Input: part model. Units: mm. Frame: model coordinates. A direction names the side the tool comes from. Coordinates: 2 decimals unless noted, no trailing zeros. Loops run counter-clockwise (first coordinate to the right, second up) from the corner with the lowest first, then second, coordinate; pieces in that order, holes last. Notation, with made-up numbers: (35.25, -2.5) - (81.25, -2.5) arc R17 ccw to (81.25, 10.5) - close; hole circle Ø5 at (51.5, 28). An arc over 180 degrees is marked (long way). Use a Markdown table: item, result. Add a question column.
1. Section query A-A on z = 0. Return the cut outline in (x, y).
2. Section query C-C on z = 3. Return the cut outline in (x, y).
3. Section query D-D on y = 6. State how many separate pieces and enclosed holes the cut face has, then the cut area to 3 significant figures.
4. Ray query, L1, parallel to X at y = 12, z = 0; L2, parallel to Z at x = -26, y = 10.5; L3, parallel to X at y = 9.5, z = -2. Return the intervals inside material, ascending. Write a range as [from, to].
5. Contact query for flat-ended pins moving along their axis: P1, Ø3, axis at y = 3, z = 4, coming from the +X side; P2, Ø6, axis at x = -11, y = 11, coming from the -Z side; P3, Ø1, axis at x = 8, z = 10.5, coming from the -Y side. Output: stop coordinate, or through.
6. Draft query along X for faces 6 (the face through (23.69, 2.6, 8.61)), 7 (the face through (0, 20, 10)), 8 (the face through (26.9, 9.9, -3.4)). Return one class per face: released by +X, released by -X, zero draft, split by the parting line, or undercut.
7. Section query B-B on x = -4.5. Return the cut outline in (y, z), then the cut area to 3 significant figures.
8. Access query for faces 1 (the face through (26.165, 2.867, 5.156)), 2 (the face through (15.671, 10.337, 11.355)), 3 (the face through (26, 0, 4)), 4 (the face through (25, 1.996, 7)), 5 (the face through (-26.73, 9.86, -3.39)). Directions: +Z, -Z, +X, -X, +Y, -Y. A direction counts if a zero-diameter tool reaches every point of the face in a straight line with its end or side. Return the directions, or none.
```python
from build123d import *

# Parameters (mm, degrees)
SKETCH_1_R               = 2.2
EXTRUDE_1_DEPTH          = 20
FILLET_1_R               = 3
SKETCH_3_W               = 5.163325916
SKETCH_3_H               = 16.003609002
CUT_EXTRUDE_2_DEPTH      = 57.596101085
FILLET_2_R               = 2
EXTRUDE_2_DEPTH          = 20
CUT_EXTRUDE_1_DEPTH      = 40.134639439
CUT_EXTRUDE_1_DEPTH_BACK = 40.134639439
SKETCH_5_W               = 17
SKETCH_5_H               = 15.6
SKETCH_5_W_2             = 3.540430575
SKETCH_5_H_2             = 6.8
CUT_EXTRUDE_3_DEPTH      = 0.4
FILLET_3_R               = 1.5


with BuildPart() as part:
    # 草图1 → 凸台-拉伸1 (new body)
    with BuildSketch(Plane(origin=(0, 0, 0), x_dir=(1, 0, 0), z_dir=(0, 1, 0))):
        with BuildLine():
            Line((-29.65627848, -2.122306442), (-22.56320207, -11))
            Line((-22.56320207, -11), (22.56320207, -11))
            Line((22.56320207, -11), (29.65627848, -2.122306442))
            ThreePointArc((29.65627848, -2.122306442), (25.48101359, 3.04182187), (27.10063693, -3.398510293))
            Line((27.10063693, -3.398510293), (21.985991405, -9.8))
            Line((21.985991405, -9.8), (-21.985991405, -9.8))
            Line((-21.985991405, -9.8), (-27.10063693, -3.398510293))
            ThreePointArc((-27.10063693, -3.398510293), (-25.48101359, 3.04182187), (-29.65627848, -2.122306442))
        make_face()
        with Locations(Location((-27, 0, 0), (0, 0, 270))):
            Circle(SKETCH_1_R, mode=Mode.SUBTRACT)
        with Locations(Location((27, 0, 0), (0, 0, 90))):
            Circle(SKETCH_1_R, mode=Mode.SUBTRACT)
    extrude(amount=EXTRUDE_1_DEPTH)

    # 圆角1
    fillet_1_edges = [part.edges().sort_by_distance(p)[0] for p in [
        (-27.10063693, 10, 3.398510293),
        (27.10063693, 10, 3.398510293),
    ]]
    fillet(fillet_1_edges, radius=FILLET_1_R)

    # 草图3 → 切除-拉伸2 (cut, through all)
    with BuildSketch(Plane(origin=(19.136124058, 0, 15.289330416), x_dir=(0.6242077770989366, 0, -0.7812583766009837), z_dir=(0.7812583766009837, 0, 0.6242077770989366))):
        with Locations((10.071947024, 9.998195499)):
            Rectangle(SKETCH_3_W, SKETCH_3_H)
    cut_extrude_2 = extrude(amount=-CUT_EXTRUDE_2_DEPTH, mode=Mode.SUBTRACT)

    # 镜向1: 切除-拉伸2 across plane
    add(cut_extrude_2.mirror(Plane(origin=(0, 0, 0), x_dir=(0, 0, 1), z_dir=(1, 0, 0))), mode=Mode.SUBTRACT)

    # 圆角2
    fillet_2_edges = [part.edges().sort_by_distance(p)[0] for p in [
        (23.342862598, 1.996390998, 9.062958581),
        (26.211335217, 18, 4.745817031),
        (26.211335217, 1.996390998, 4.745817031),
        (23.342862598, 18, 9.062958581),
        (-23.342862598, 18, 9.062958581),
        (-26.211335217, 1.996390998, 4.745817031),
        (-26.211335217, 18, 4.745817031),
        (-23.342862598, 1.996390998, 9.062958581),
    ]]
    fillet(fillet_2_edges, radius=FILLET_2_R)

    # 草图4 → 凸台-拉伸2 (add)
    with BuildSketch(Plane(origin=(0, 20, 0), x_dir=(1, 0, 0), z_dir=(0, 1, 0))):
        Polygon((-22.56320207, -11), (-22.003917898, -11.7), (-16.284224925, -11.7), (-15.040430575, -11), align=None)
        Polygon((15.040430575, -11), (22.56320207, -11), (22.003917898, -11.7), (16.284224925, -11.7), align=None)
    extrude(amount=-EXTRUDE_2_DEPTH)

    # 草图2 → 切除-拉伸1 (cut, two sides: drawn at the far end of the back side and taken through both)
    with BuildSketch(Plane.XY.offset(11).offset(-CUT_EXTRUDE_1_DEPTH_BACK)):
        Polygon((-19.273176969, 0), (-17.2479344, 0.4), (17.2479344, 0.4), (19.273176969, 0), align=None)
    extrude(amount=CUT_EXTRUDE_1_DEPTH + CUT_EXTRUDE_1_DEPTH_BACK, mode=Mode.SUBTRACT)

    # 草图5 → 切除-拉伸3 (cut)
    with BuildSketch(Plane.XY.offset(11)):
        with Locations((0, 10.2)):
            Rectangle(SKETCH_5_W, SKETCH_5_H)
        with Locations((-11.770215288, 14.6)):
            Rectangle(SKETCH_5_W_2, SKETCH_5_H_2)
        with Locations((11.770215288, 14.6)):
            Rectangle(SKETCH_5_W_2, SKETCH_5_H_2)
        with Locations((-11.770215288, 5.8)):
            Rectangle(SKETCH_5_W_2, SKETCH_5_H_2)
        with Locations((11.770215288, 5.8)):
            Rectangle(SKETCH_5_W_2, SKETCH_5_H_2)
    extrude(amount=-CUT_EXTRUDE_3_DEPTH, mode=Mode.SUBTRACT)

    # 圆角3
    fillet_3_edges = [part.edges().sort_by_distance(p)[0] for p in [
        (13.540430575, 2.4, 10.8),
        (10, 2.4, 10.8),
        (10, 9.2, 10.8),
        (13.540430575, 9.2, 10.8),
        (-13.540430575, 2.4, 10.8),
        (-13.540430575, 9.2, 10.8),
        (-10, 9.2, 10.8),
        (-10, 2.4, 10.8),
        (13.540430575, 18, 10.8),
        (13.540430575, 11.2, 10.8),
        (10, 11.2, 10.8),
        (10, 18, 10.8),
        (-10, 18, 10.8),
        (-10, 11.2, 10.8),
        (-13.540430575, 11.2, 10.8),
        (-13.540430575, 18, 10.8),
        (8.5, 18, 10.8),
        (8.5, 2.4, 10.8),
        (-8.5, 2.4, 10.8),
        (-8.5, 18, 10.8),
    ]]
    fillet(fillet_3_edges, radius=FILLET_3_R)


solid = part.part
```
Resolved:
| question | item | result |
|---|---|---|
| 1 | outline | (-30.4, 0) - (-29.2, 0) - (-29.2, 20) - (-30.4, 20) - close; (-24.8, 0) - (-23.6, 0) - (-23.6, 20) - (-24.8, 20) - close; (23.6, 0) - (24.8, 0) - (24.8, 20) - (23.6, 20) - close; (29.2, 0) - (30.4, 0) - (30.4, 20) - (29.2, 20) - close |
| 2 | outline | (-28.96, 0) - (-25.03, 0) - (-25.03, 20) - (-28.96, 20) - close; (25.03, 0) - (28.96, 0) - (28.96, 20) - (25.03, 20) - close |
| 3 | separate pieces | 3 |
| 3 | enclosed holes | 2 |
| 3 | area | 109 mm² |
| 4 | L1 | [-30.4, -29.2], [-24.8, -23.6], [23.6, 24.8], [29.2, 30.4] |
| 4 | L2 | [-3.25, -1.96], [1.96, 4.58] |
| 4 | L3 | [-29.75, -27.92], [-26.08, -24.25], [24.25, 26.08], [27.92, 29.75] |
| 5 | P1 | x = 29.35 |
| 5 | P2 | z = 9.8 |
| 5 | P3 | y = 0.4 |
| 6 | face 6 | released by +X |
| 6 | face 7 | zero draft |
| 6 | face 8 | undercut |
| 7 | outline | (0.4, 9.8) - (20, 9.8) - (20, 11) - (18, 11) - (18, 10.6) - (2.4, 10.6) - (2.4, 11) - (0.4, 11) - close |
| 7 | area | 17.3 mm² |
| 8 | face 1 | +Z |
| 8 | face 2 | +Z, +Y, -Y |
| 8 | face 3 | +Z, -Z, +X, -X, -Y |
| 8 | face 4 | none |
| 8 | face 5 | +Y, -Y |
